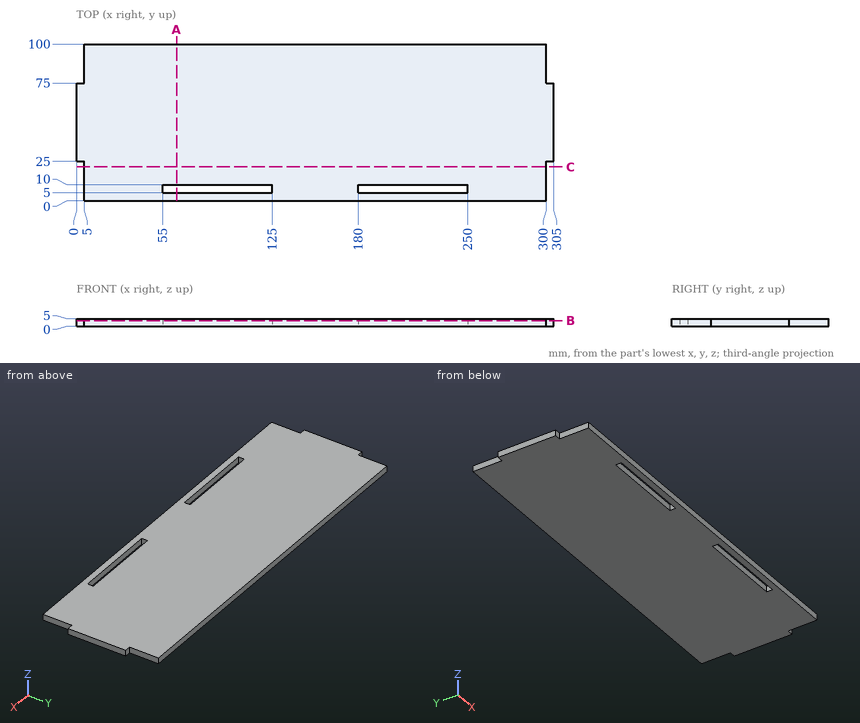
Verification items for this drawing (mm, ordinates from the low corner). Round coordinates to 2 decimals unless told otherwise and drop trailing zeros. Loops run counter-clockwise (first coordinate to the right, second up) from the corner with the lowest first, then second, coordinate; pieces in that order, holes last. Notation, with made-up numbers: M 85.25,18 L 93.25,18 A12 cw 93.25,26 Z; hole C 37,77.25 d10. An arc over 180 degrees is marked long. Answer as a JSON object with one key per item and string values.
1. Gauge pin test, flat ends, axial feed: P1, Ø1.5, axis at y = 8.5, z = 2.5, coming from the +X side; P2, Ø2.5, axis at y = 13.5, z = 3.5, coming from the -X side; P3, Ø1.5, axis at x = 1.5, z = 2, coming from the -Y side. Record the tip position at first contact, or that the pin passes through.
Reply:
{"P1": "stops at x = 300", "P2": "stops at x = 5", "P3": "stops at y = 25"}
2. Section check C-C (y = 21.5). Record the boundary of the cut face in (x, z).
Reply:
{"outline": "M 5,0 L 300,0 L 300,5 L 5,5 Z"}
3. Section check A-A (x = 64). Record the boundary of the cut face in (y, z), plus the area to 3 significant figures.
Reply:
{"outline": "M 0,0 L 5,0 L 5,5 L 0,5 Z; M 10,0 L 100,0 L 100,5 L 10,5 Z", "area": "475 mm²"}
4. Scan lines: line 1 (X direction, y = 5.5, z = 4.65); line 2 (Y direction, x = 100, z = 0.6); line 3 (X direction, y = 93.5, z = 3.6). Record each from-to range of solid material in increasing order.
Reply:
{"line 1": "x = 5 to 55, 125 to 180, 250 to 300", "line 2": "y = 0 to 5, 10 to 100", "line 3": "x = 5 to 300"}
5. Section check B-B (z = 3.6). Record the boundary of the cut face in (x, y).
Reply:
{"outline": "M 0,25 L 5,25 L 5,0 L 300,0 L 300,25 L 305,25 L 305,75 L 300,75 L 300,100 L 5,100 L 5,75 L 0,75 Z; hole M 55,5 L 125,5 L 125,10 L 55,10 Z; hole M 180,5 L 250,5 L 250,10 L 180,10 Z"}
